CAD build for the part. Positions are in the model's coordinates, mm. A direction names the side the tool comes from. Round coordinates to 2 decimals unless told otherwise and drop trailing zeros. Write each loop counter-clockwise with the first axis right and the second up, starting at its lowest first coordinate (ties: lowest second). Pieces come first, ordered by that corner, then holes. Notation, with made-up numbers: (37, 87.25) - (47, 87.25) arc R34 cw to (47, 120.25) - close; hole circle Ø8 at (-22.75, -10.5). An arc over 180 degrees is marked (long way). Answer in a Markdown table with one row per item.
```python
from build123d import *

# Parameters (mm, degrees)
SKETCH1_R               = 5
BOSS_EXTRUDE1_DEPTH     = 5
SKETCH2_R               = 5.5
BOSS_EXTRUDE2_DEPTH     = 0.4
CUT_EXTRUDE1_DEPTH      = 6.4
SKETCH5_R               = 8
CUT_EXTRUDE2_DEPTH      = 6.5
CUT_EXTRUDE2_DEPTH_BACK = 6.5
CHAMFER4_SIZE           = 1
CHAMFER4_SIZE2          = 0.383864035
SKETCH7_W               = 5
SKETCH7_H               = 6.5
BOSS_EXTRUDE4_DEPTH     = 1.5


with BuildPart() as part:
    # Sketch1 → Boss-Extrude1 (new body)
    with BuildSketch(Plane(origin=(0, 0, 0), x_dir=(1, 0, 0), z_dir=(0, 1, 0))):
        Circle(SKETCH1_R)
    extrude(amount=BOSS_EXTRUDE1_DEPTH)

    # Sketch2 → Boss-Extrude2 (add)
    with BuildSketch(Plane(origin=(0, 5, 0), x_dir=(1, 0, 0), z_dir=(0, 1, 0))):
        Circle(SKETCH2_R)
    extrude(amount=BOSS_EXTRUDE2_DEPTH)

    # Sketch4 → Cut-Extrude1 (cut, through all)
    with BuildSketch(Plane(origin=(0, 5.4, 0), x_dir=(1, 0, 0), z_dir=(0, 1, 0))):
        with BuildLine():
            Line((2.295250379, 1.5), (2.295250379, -1.5))
            ThreePointArc((2.295250379, -1.5), (0, -3.795250379), (-2.295250379, -1.5))
            Line((-2.295250379, -1.5), (-2.295250379, 1.5))
            ThreePointArc((-2.295250379, 1.5), (0, 3.795250379), (2.295250379, 1.5))
        make_face()
    extrude(amount=-CUT_EXTRUDE1_DEPTH, mode=Mode.SUBTRACT)

    # Sketch5 → Cut-Extrude2 (cut, two sides)
    with BuildSketch(Plane(origin=(0, 0, 0), x_dir=(0, 0, -1), z_dir=(1, 0, 0))) as cut_extrude2_sk:
        with Locations((0, -3)):
            Circle(SKETCH5_R)
    extrude(amount=CUT_EXTRUDE2_DEPTH, mode=Mode.SUBTRACT)
    extrude(cut_extrude2_sk.sketch, amount=-CUT_EXTRUDE2_DEPTH_BACK, mode=Mode.SUBTRACT)

    # Chamfer4
    chamfer4_edges = [part.edges().sort_by_distance(p)[0] for p in [
        (0, 5.4, -3.795250379),
        (-2.295250379, 5.4, 0),
        (0, 5.4, 3.795250379),
        (2.295250379, 5.4, 0),
    ]]
    chamfer4_side = [part.faces().sort_by_distance(p)[0] for p in [
        (-5.344436508, 5.4, 0),
    ]]
    chamfer(chamfer4_edges, length=CHAMFER4_SIZE, length2=CHAMFER4_SIZE2, reference=chamfer4_side[0])

    # Sketch7 → Boss-Extrude4 (add)
    with BuildSketch(Plane(origin=(0, 5.4, 0), x_dir=(1, 0, 0), z_dir=(0, 1, 0))):
        with Locations((0, 7.75)):
            Rectangle(SKETCH7_W, SKETCH7_H)
        with Locations((0, -7.75)):
            Rectangle(SKETCH7_W, SKETCH7_H)
    extrude(amount=-BOSS_EXTRUDE4_DEPTH)


solid = part.part
```
Q1. Drill centre lines: line 1 (Z direction, x = 0, y = 4.5); line 2 (X direction, y = 4.05, z = 6.5); line 3 (Y direction, x = -1, z = 9.25). Where is each one in solid material? Low to high.
Computed:
| item | result |
|---|---|
| line 1 | z = -11 to -3.8, 3.8 to 11 |
| line 2 | x = -2.5 to 2.5 |
| line 3 | y = 3.9 to 5.4 |
Q2. Saw through at A-A on x = 0. List the corners of the cut face in (y, z) (3 decimals), then the cut area to 3 significant figures.
Computed:
| item | result |
|---|---|
| outline | (3.245, -5) - (3.9, -5) - (3.9, -11) - (5.4, -11) - (5.4, -4.5) - (5.287, -4.5) - (5.016, -3.795) - (4.042, -3.795) arc R8 cw to start; (3.245, 5) arc R8 cw to (4.042, 3.795) - (5.016, 3.795) - (5.287, 4.5) - (5.4, 4.5) - (5.4, 11) - (3.9, 11) - (3.9, 5) - close |
| area | 21.8 mm2 |
Q3. Saw through at B-B on y = 4.65. List the corners of the cut face in (x, z).
Computed:
| item | result |
|---|---|
| outline | (-4.42, -2.34) arc R5 ccw to (-2.18, -4.5) - (-2.5, -4.5) - (-2.5, -11) - (2.5, -11) - (2.5, -4.5) - (2.18, -4.5) arc R5 ccw to (4.42, -2.34) - (2.14, -2.34) arc R2.3 cw to (-2.14, -2.34) - close; (-4.42, 2.34) - (-2.14, 2.34) arc R2.3 cw to (2.14, 2.34) - (4.42, 2.34) arc R5 ccw to (2.18, 4.5) - (2.5, 4.5) - (2.5, 11) - (-2.5, 11) - (-2.5, 4.5) - (-2.18, 4.5) arc R5 ccw to start |
Q4. 3-axis set-ups, long thin cutter, end or side, ignore diameter. For faces 4 (the flat face through (2.788, 5.205, -0.021)), 5 (the cylindrical face through (0.05, 4.644, 3.795)), 6 (the cylindrical face through (3, 5, 0)): which of +Z, -Z, +X, -X, +Y, -Y reach the whole face in a straight line?
Computed:
| item | result |
|---|---|
| face 4 | +Y |
| face 5 | +Y, -Y |
| face 6 | +X, -X, -Y |
Q5. Flat gauge pins, fed straight in: pin 1 (1.5 mm diameter, centred on x = 2.5, z = -1, fed in from -Y); pin 2 (6 mm diameter, centred on x = -1.5, z = 8, fed in from -Y); pin 3 (1.2 mm diameter, centred on y = 5, z = -8, fed in from -X); pin 4 (4 mm diameter, centred on x = -1, z = -3, fed in from +Y). Where does each tip first touch, or does it go through?
Computed:
| item | result |
|---|---|
| pin 1 | stops at y = 4.81 |
| pin 2 | stops at y = 3.9 |
| pin 3 | stops at x = -2.5 |
| pin 4 | stops at y = 5.4 |
Q6. Pull direction X, two halves, no side cores. Call faces 1 (the cylindrical face through (-0.05, 4.644, -3.795)), 2 (the flat face through (0, 3.9, 8)), 3 (the cylindrical face through (5.5, 5.2, 0.1)): released by +X, released by -X, zero draft, split by the parting line, or undercut.
Computed:
| item | result |
|---|---|
| face 1 | undercut |
| face 2 | zero draft |
| face 3 | released by +X |
